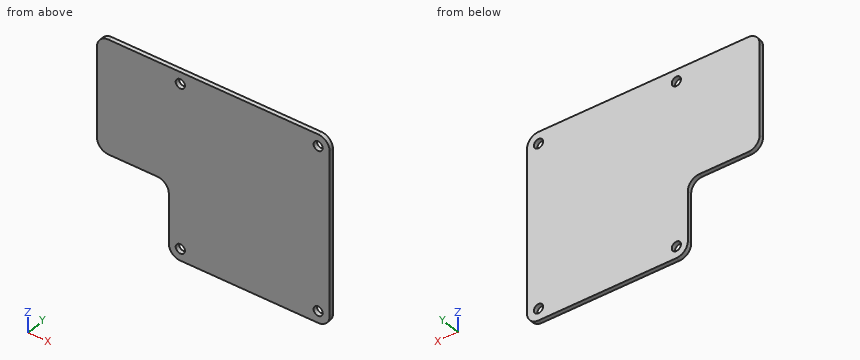
```python
from build123d import *

# Parameters (mm, degrees)
SKETCH1_R           = 1.6
BOSS_EXTRUDE1_DEPTH = 1.5


with BuildPart() as part:
    # Sketch1 → Boss-Extrude1 (new body)
    with BuildSketch(Plane(origin=(0, 0, 0), x_dir=(1, 0, 0), z_dir=(0, 1, 0))):
        with BuildLine():
            Line((-8, 35), (-25, 35))
            ThreePointArc((-25, 35), (-27.828427125, 33.828427125), (-29, 31))
            Line((-29, 31), (-29, 0))
            ThreePointArc((-29, 0), (-27.828427125, -2.828427125), (-25, -4))
            Line((-25, -4), (-8, -4))
            Line((-8, -4), (48, -4))
            ThreePointArc((48, -4), (50.828427125, -2.828427125), (52, 0))
            Line((52, 0), (52, 56))
            ThreePointArc((52, 56), (50.828427125, 58.828427125), (48, 60))
            Line((48, 60), (0, 60))
            ThreePointArc((0, 60), (-2.828427125, 58.828427125), (-4, 56))
            Line((-4, 56), (-4, 39))
            ThreePointArc((-4, 39), (-5.171572875, 36.171572875), (-8, 35))
        make_face()
        with Locations((0, 56)):
            Circle(SKETCH1_R, mode=Mode.SUBTRACT)
        with Locations((48, 56)):
            Circle(SKETCH1_R, mode=Mode.SUBTRACT)
        with Locations((48, 0)):
            Circle(SKETCH1_R, mode=Mode.SUBTRACT)
        Circle(SKETCH1_R, mode=Mode.SUBTRACT)
    extrude(amount=BOSS_EXTRUDE1_DEPTH)


solid = part.part
```
Check sheet for the modelled part. Datum: model origin and axes. Units: mm. Give positions to 0.01 mm unless a question says otherwise; leave off trailing zeros. Write each loop counter-clockwise with the first axis right and the second up, starting at its lowest first coordinate (ties: lowest second). Pieces come first, ordered by that corner, then holes.
Item 1: Scan lines: L1, parallel to X at y = 0.4, z = 0; L2, parallel to X at y = 0.95, z = -56; L3, parallel to Z at x = 48, y = 1. Record each from-to range of solid material in increasing order.
Item 2: Cross-section at A-A (y = 0.25). Enter the section's corners in (x, z).
Item 3: Cross-section at B-B (x = -11). Enter the section's corners in (y, z).
Report:
1. L1: x = -29 to -1.6, 1.6 to 46.4, 49.6 to 52
1. L2: x = -4 to -1.6, 1.6 to 46.4, 49.6 to 52
1. L3: z = -60 to -57.6, -54.4 to -1.6, 1.6 to 4
2. outline: (-29, -31) arc R4 ccw to (-25, -35) - (-8, -35) arc R4 cw to (-4, -39) - (-4, -56) arc R4 ccw to (0, -60) - (48, -60) arc R4 ccw to (52, -56) - (52, 0) arc R4 ccw to (48, 4) - (-25, 4) arc R4 ccw to (-29, 0) - close; hole circle Ø3.2 at (0, -56); hole circle Ø3.2 at (0, 0); hole circle Ø3.2 at (48, -56); hole circle Ø3.2 at (48, 0)
3. outline: (0, -35) - (1.5, -35) - (1.5, 4) - (0, 4) - close
